Geometry check sheet. Reference: the model listing, model coordinates, mm. Give positions to 0.01 mm unless a question says otherwise; leave off trailing zeros. Order: outer loops, then holes, each group sorted by start corner. A loop starts at its lowest first (then second) coordinate and runs counter-clockwise, first axis right, second up.
from build123d import *

# Parameters (mm, degrees)
BOSS_EXTRUDE1_DEPTH      = 1.5
M3_CLEARANCE_HOLE1_D     = 3.2
M3_CLEARANCE_HOLE1_DEPTH = 3


with BuildPart() as part:
    # Sketch1 → Boss-Extrude1 (new body, symmetric)
    with BuildSketch(Plane(origin=(0, 0, 0), x_dir=(1, 0, 0), z_dir=(0, 1, 0))):
        with BuildLine():
            Line((-5, 6), (5, 6))
            ThreePointArc((5, 6), (11, 0), (5, -6))
            Line((5, -6), (-5, -6))
            ThreePointArc((-5, -6), (-11, 0), (-5, 6))
        make_face()
    extrude(amount=BOSS_EXTRUDE1_DEPTH, both=True)

    # M3 Clearance Hole1
    with Locations(Plane(origin=(0, 1.5, 0), x_dir=(1, 0, 0), z_dir=(0, 1, 0))):
        with Locations((-5, 0), (5, 0)):
            Hole(M3_CLEARANCE_HOLE1_D / 2, depth=M3_CLEARANCE_HOLE1_DEPTH)


solid = part.part
Item 1: Scan lines: L1, parallel to X at y = -1, z = 1.25; L2, parallel to Z at x = -5, y = -0.8; L3, parallel to Z at x = -6, y = 0.1. Record each from-to range of solid material in increasing order.
Reported:
L1: x = -10.87 to -6, -4 to 4, 6 to 10.87
L2: z = -6 to -1.6, 1.6 to 6
L3: z = -5.92 to -1.25, 1.25 to 5.92
Item 2: Sectioned sample at A-A (z = 0). Enter the section's corners in (x, y), and give its area (3 significant figures).
Reported:
outline: (-11, -1.5) - (-6.6, -1.5) - (-6.6, 1.5) - (-11, 1.5) - close; (-3.4, -1.5) - (3.4, -1.5) - (3.4, 1.5) - (-3.4, 1.5) - close; (6.6, -1.5) - (11, -1.5) - (11, 1.5) - (6.6, 1.5) - close
area: 46.8 mm2
Item 3: Sectioned sample at C-C (x = -8.5). Enter the section's corners in (y, z), and give its area (3 significant figures).
Reported:
outline: (-1.5, -4.87) - (1.5, -4.87) - (1.5, 4.87) - (-1.5, 4.87) - close
area: 29.2 mm2
Item 4: Sectioned sample at B-B (y = 0.45). Enter the section's corners in (x, z).
Reported:
outline: (-5, -6) - (5, -6) arc R6 ccw to (5, 6) - (-5, 6) arc R6 ccw to start; hole circle Ø3.2 at (-5, 0); hole circle Ø3.2 at (5, 0)
Item 5: Sectioned sample at D-D (z = -2.5). Enter the section's corners in (x, y).
Reported:
outline: (-10.45, -1.5) - (10.45, -1.5) - (10.45, 1.5) - (-10.45, 1.5) - close
Item 6: Gauge pin test, flat ends, axial feed: pin 1 (5 mm diameter, centred on x = 5, z = 0, fed in from -Y); pin 2 (1.9 mm diameter, centred on x = -5, z = 0, fed in from +Y); pin 3 (1.5 mm diameter, centred on y = -1, z = -1.5, fed in from +X). Record the tip position at first contact, or that the pin passes through.
Reported:
pin 1: stops at y = -1.5
pin 2: passes through
pin 3: stops at x = 10.95
Item 7: Draft check along X on faces 1 (the cylindrical face through (6.6, -0.02, -0.07)), 2 (the flat face through (0, 0, 6)), 3 (the cylindrical face through (-3.4, -0.02, -0.07)), 4 (the cylindrical face through (-11, 0, 0)). Enter one of: released by +X, released by -X, zero draft, split by the parting line, or undercut.
Reported:
face 1: undercut
face 2: zero draft
face 3: undercut
face 4: released by -X
